from build123d import *

# Parameters (mm, degrees)
IZIM1_R            = 10
TABAN_FLAN_1_DEPTH = 15


# Sheet-metal steps are written as plain solids
with BuildPart() as part:
    # Çizim1 → Taban-Flanş1 (new body)
    with BuildSketch(Plane.XY):
        with BuildLine():
            Line((-154.698643159, 156.857538138), (-192.024974986, 22.709348381))
            ThreePointArc((-192.024974986, 22.709348381), (85.964362875, -3.168316981), (362.465125286, 35.497610073))
            ThreePointArc((362.465125286, 35.497610073), (349.092339052, 102.938005803), (327.738170112, 168.291183666))
            ThreePointArc((327.738170112, 168.291183666), (318.781629996, 177.759788443), (306.201680975, 181.168449454))
            ThreePointArc((306.201680975, 181.168449454), (89.247279864, 151.970973974), (-129.053786306, 168.291183666))
            ThreePointArc((-129.053786306, 168.291183666), (-143.060537772, 165.230713571), (-154.698643159, 156.857538138))
        make_face()
        with Locations((-112.183904076, 131.277032831)):
            Circle(IZIM1_R, mode=Mode.SUBTRACT)
        with Locations((21.040997306, 116.885172221)):
            Circle(IZIM1_R, mode=Mode.SUBTRACT)
        with Locations((154.983782422, 120.800566875)):
            Circle(IZIM1_R, mode=Mode.SUBTRACT)
        with Locations((287.140513745, 142.950022083)):
            Circle(IZIM1_R, mode=Mode.SUBTRACT)
    extrude(amount=-TABAN_FLAN_1_DEPTH)


solid = part.part
For this review, take the finished solid that the model builds, in its own axes (mm). Round coordinates to 2 decimals unless told otherwise and drop trailing zeros. Order: outer loops, then holes, each group sorted by start corner. A loop starts at its lowest first (then second) coordinate and runs counter-clockwise, first axis right, second up. Notation, with made-up numbers: M 15.5,-40 L 71.5,-40 A16 ccw 71.5,-32 Z; hole C 80,-16.75 d2. An arc over 180 degrees is marked long. Write each question's results on one line, items separated by ' | '. Start each with the question number.
1. Add section A-A (z = -11.75). State the section outline as (x, y) points.
2. Add section C-C (y = 88). State the section outline as (x, z) points.
3. Add section B-B (x = 85). State the section outline as (y, z) points, then the cut area to 3 significant figures.
4. Clearance check with flat-ended pins moving along their axes: pin 1 Ø4 at (x, y) = (219.5, 37.5) entering from +Z; pin 2 Ø8 at (x, z) = (244, -11.5) entering from -Y; pin 3 Ø5 at (y, z) = (157, -4.5) entering from +X; pin 4 Ø4 at (x, z) = (-93, -10) entering from -Y. State where each tip first meets the part, or that it passes through.
5. To check wall thickness, follow L1, parallel to X at y = 120, z = -12; L2, parallel to Y at x = -109, z = -9.5; L3, parallel to X at y = 102, z = -12.5. State the ranges of each line that lie inside material, in increasing order. Write a range as [from, to].
6. Draft analysis for pull direction X (two halves, no side actions). For faces 1 (the face through (144.993, 121.24, -7.395)), 2 (the face through (81, 90, -15)), 3 (the face through (-142.9, 165.3, -7.4)), state which applies: pulls with the +X half, pulls with the -X half, needs draft (parallel to the pull), parting line crosses it, or undercut.
Output values:
1) outline: M -192.02,22.71 A1207.35 ccw 362.47,35.5 A572.99 ccw 327.74,168.29 A24.06 ccw 306.2,181.17 A1052.35 cw -129.05,168.29 A35.34 ccw -154.7,156.86 Z; hole C -112.18,131.28 d20; hole C 21.04,116.89 d20; hole C 154.98,120.8 d20; hole C 287.14,142.95 d20
2) outline: M -173.86,-15 L 352.79,-15 L 352.79,0 L -173.86,0 Z
3) outline: M -3.19,-15 L 151.85,-15 L 151.85,0 L -3.19,0 Z | area: 2,330 mm^2
4) pin 1: z = 0 | pin 2: y = 10.29 | pin 3: x = 332.98 | pin 4: y = 5.76
5) L1: [-164.95, 11.54], [30.54, 145.02], [164.95, 344.35] | L2: [8.13, 121.8], [140.76, 164.87] | L3: [-169.96, 349.34]
6) face 1: undercut | face 2: needs draft | face 3: pulls with the -X half
